Geometry check sheet. Reference: the model listing, model coordinates, mm. Round coordinates to 2 decimals unless told otherwise and drop trailing zeros. Write each loop counter-clockwise with the first axis right and the second up, starting at its lowest first coordinate (ties: lowest second). Pieces come first, ordered by that corner, then holes. Notation, with made-up numbers: M 77,-7.5 L 83,-7.5 A16 cw 83,6.5 Z; hole C 89.25,18 d8. An arc over 180 degrees is marked long. One line per item, written item: value. Start each with the question number.
1. Scan lines: probe 1 along Z at (x, y) = (6, 82.5); probe 2 along X at (y, z) = (287, 2.5) (3 decimals); probe 3 along Y at (x, z) = (-30.5, 2). Record each from-to range of solid material in increasing order. Write a range as [from, to].
2. Section check A-A (x = 9). Record the boundary of the cut face in (y, z).
3. Depth check by flat-ended pin: P1, Ø4.5, axis at x = 0, y = 327.025, coming from the +Z side; P2, Ø4, axis at x = 0, y = 276.225, coming from the -Z side; P3, Ø3, axis at x = 0, y = 85.54, coming from the +Z side; P4, Ø4, axis at y = 155.5, z = 1.5, coming from the +X side (3 decimals). Enter the tip coordinate at first touch or a pass-through.
from build123d import *

# Parameters (mm, degrees)
BOSS_EXTRUDE1_DEPTH                             = 4.826
SKETCH2_R                                       = 33.3375
CUT_EXTRUDE1_DEPTH                              = 347.01033464659696
FILLET1_R                                       = 25.400000000000002
LPATTERN2_COUNT                                 = 19
LPATTERN2_PITCH                                 = 12.7
CSK_FOR_M3_FLAT_HEAD_MACHINE_SCREW1_D           = 3.3
CSK_FOR_M3_FLAT_HEAD_MACHINE_SCREW1_CSINK_D     = 6.35
CSK_FOR_M3_FLAT_HEAD_MACHINE_SCREW1_CSINK_ANGLE = 90
CIRPATTERN1_COUNT                               = 6
BOSS_EXTRUDE2_DEPTH                             = 7
BOSS_EXTRUDE2_DEPTH_BACK                        = 5.326


with BuildPart() as part:
    # Sketch1 → Boss-Extrude1 (new body)
    with BuildSketch(Plane.XY):
        with BuildLine():
            Line((15.875, 89.25133784449143), (15.875, 327.02500000000003))
            ThreePointArc((15.875, 327.02500000000003), (3.68e-15, 342.90000000000003), (-15.875, 327.02500000000003))
            Line((-15.875, 327.02500000000003), (-15.875, 89.25133784449143))
            ThreePointArc((-15.875, 89.25133784449143), (-8.46e-15, 7.11e-15), (15.875, 89.25133784449143))
        make_face()
    extrude(amount=BOSS_EXTRUDE1_DEPTH)

    # Sketch2 → Cut-Extrude1 (cut, through all)
    with BuildSketch(Plane.XY.offset(4.826)):
        with Locations((0, 46.0375)):
            Circle(SKETCH2_R)
    extrude(amount=-CUT_EXTRUDE1_DEPTH, mode=Mode.SUBTRACT)

    # Fillet1
    fillet1_edges = [part.edges().sort_by_distance(p)[0] for p in [
        (-15.874999999999998, 89.25133784449142, 2.413),
        (15.875000000000002, 89.25133784449145, 2.413),
    ]]
    fillet(fillet1_edges, radius=FILLET1_R)

    # Sketch4 → 8-32 Tapped Hole1 (revolve, cut)
    with BuildSketch(Plane(origin=(2.71e-15, 327.02500000000003, 4.826), x_dir=(0, -1, 0), z_dir=(1, 0, 0))):
        Polygon((0, 0), (-2.87e-15, 11.705806461184395), (1.7271999999999874, 10.667999999999997), (1.7271999999999894, -1.34e-15), align=None)
    f_8_32_tapped_hole1 = revolve(axis=Axis((2.71e-15, 327.02500000000003, 11.175999999999991), (0, 0, -1)), mode=Mode.SUBTRACT)

    # LPattern2: 8-32 Tapped Hole1 ×19
    with Locations(*[(0, -i * LPATTERN2_PITCH, 0) for i in range(1, LPATTERN2_COUNT)]):
        add(f_8_32_tapped_hole1, mode=Mode.SUBTRACT)

    # CSK for M3 Flat Head Machine Screw1 (through all)
    with Locations(Plane(origin=(0, 0, 0), x_dir=(-1, 0, 0), z_dir=(0, 0, -1))):
        with Locations((0, 85.537499994)):
            csk_for_m3_flat_head_machine_screw1 = CounterSinkHole(CSK_FOR_M3_FLAT_HEAD_MACHINE_SCREW1_D / 2, CSK_FOR_M3_FLAT_HEAD_MACHINE_SCREW1_CSINK_D / 2, counter_sink_angle=CSK_FOR_M3_FLAT_HEAD_MACHINE_SCREW1_CSINK_ANGLE)

    # CirPattern1: CSK for M3 Flat Head Machine Screw1 ×6 about axis
    cirpattern1_axis = Axis((4.857e-14, 46.037500000000016, 0), (0, 0, 1))
    for i in range(1, CIRPATTERN1_COUNT):
        add(csk_for_m3_flat_head_machine_screw1.rotate(cirpattern1_axis, i * 360 / CIRPATTERN1_COUNT), mode=Mode.SUBTRACT)

    # Sketch10 → Boss-Extrude2 (add, two sides: drawn at the far end of the back side and taken through both)
    with BuildSketch(Plane(origin=(0, 0, 0), x_dir=(-1, 0, 0), z_dir=(0, 0, -1)).offset(-BOSS_EXTRUDE2_DEPTH_BACK)):
        with BuildLine():
            Line((40.89851071944933, 24.900725714856833), (43.56363224338846, 23.52336328519776))
            ThreePointArc((43.56363224338846, 23.52336328519776), (33.850837788631225, 10.557968051878454), (20.443654867474322, 1.4647125405018753))
            Line((20.443654867474322, 1.4647125405018753), (19.192959693323495, 4.19157182938271))
            ThreePointArc((19.192959693323495, 4.19157182938271), (31.77992240008383, 12.728523154491043), (40.89851071944933, 24.900725714856833))
        make_face()
    extrude(amount=BOSS_EXTRUDE2_DEPTH + BOSS_EXTRUDE2_DEPTH_BACK)

    # Sweep2: sweep along a curve in space
    with BuildLine() as sweep2_path:
        ThreePointArc((-40.89851071944929, 24.900725714856783, 1.73e-15), (-31.779922400083795, 12.728523154491036, 9.2e-16), (-19.192959693323488, 4.191571829382735, 0))
    # Sketch12 → Sweep2 (sweep)
    with BuildSketch(Plane(origin=(-17.445500140285052, 8.001514022037082, 0), x_dir=(0, 0, -1), z_dir=(0.908953096293619, -0.41689839138361184, 0))):
        with BuildLine():
            Line((0, -4.191571829382516), (3.5, -4.191571829382516))
            ThreePointArc((3.5, -4.191571829382516), (1.4844355629253627, -3.6563095942631314), (0, -2.1915718293825166))
            Line((0, -2.1915718293825166), (0, -4.191571829382516))
        make_face()
    sweep(path=sweep2_path.line)


solid = part.part
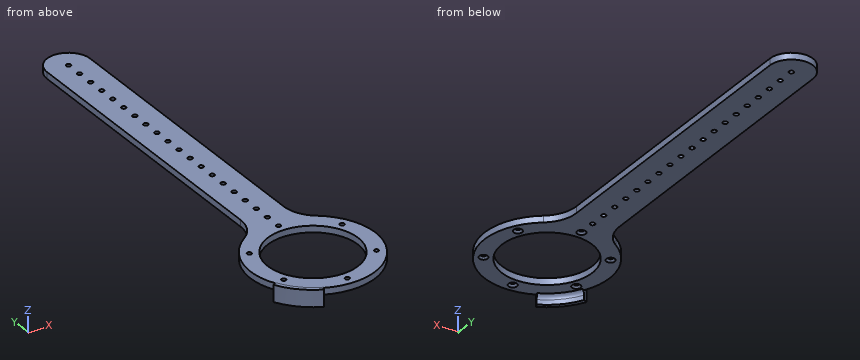
Result sheet:
1. probe 1: z = [0, 4.83]
1. probe 2: x = [-15.875, 15.875]
1. probe 3: y = [7.64, 32.58], [59.5, 80.52]
2. outline: M 0.89,0 L 13.94,0 L 13.94,4.83 L 0.89,4.83 Z; M 78.14,0 L 340.1,0 L 340.1,4.83 L 78.14,4.83 Z
3. P1: stops at z = 4.83
3. P2: stops at z = 0
3. P3: passes through
3. P4: stops at x = 15.875
